The listing builds one solid part. Answer for the finished solid, in the listing's coordinates (mm). Face numbers are marked on the shaded views. Give positions to 0.01 mm unless a question says otherwise; leave off trailing zeros. Order: outer loops, then holes, each group sorted by start corner. A loop starts at its lowest first (then second) coordinate and runs counter-clockwise, first axis right, second up. Notation, with made-up numbers: (-28.5, 67) - (14.5, 67) arc R30 ccw to (14.5, 90) - close; hole circle Ø10 at (27.5, -1.5). An arc over 180 degrees is marked (long way). Answer as a JSON object with one key per item and string values. Group by question number.
Q1. The mould has two halves that part along Y. Classify the marked faces 1, 2, 3 and 4: released by +Y, released by -Y, zero draft, split by the parting line, or undercut.
Q2. Consider line 1 (Y direction, x = -70, z = -7); line 2 (Y direction, x = 17, z = 3); line 3 (Y direction, x = 7, z = 6.75) (1 decimal). Determine where each line is inside the solid, lowest interval first.
Q3. A cutting plane is placed at B-B, the plane y = -36. Give the vertices of the cut face in (x, z), and give its area (3 significant figures).
Q4. Given pin 1 (1.5 mm diameter, centred on y = 1.5, z = 0, fed in from +X); pin 2 (1.5 mm diameter, centred on x = -60.5, z = 5, fed in from -Y); pin 3 (1.5 mm diameter, centred on x = -41.5, z = -2, fed in from -Y), each flat-ended and moving along its own axis, determine where each tip first touches the part or whether it passes through.
Q5. A cutting plane is placed at A-A, the plane x = -70. Give the vertices of the cut face in (y, z).
Q6. A cutting plane is placed at C-C, the plane y = 0. Give the vertices of the cut face in (x, z).
Q7. A cutting plane is placed at D-D, the plane z = 5.5. Give the vertices of the cut face in (x, y) (3 decimals), and give its area (3 significant figures).
from build123d import *

# Parameters (mm, degrees)
SKETCH1_R           = 7.5
SKETCH1_R_2         = 15
BOSS_EXTRUDE1_DEPTH = 15


with BuildPart() as part:
    # Sketch1 → Boss-Extrude1 (new, symmetric)
    with BuildSketch(Plane.XY):
        with BuildLine():
            ThreePointArc((13.416465379, -41.130588018), (27.104825758, -44.598880973), (30.614150003, -30.920982406))
            ThreePointArc((30.614150003, -30.920982406), (23.463789692, -15.074619609), (19.905470006, 1.94223167))
            ThreePointArc((19.905470006, 1.94223167), (9.291872744, 17.710479974), (-9.714285714, 17.482352618))
            ThreePointArc((-9.714285714, 17.482352618), (-37.932007586, 8.122402385), (-67.619047619, 9.712418121))
            ThreePointArc((-67.619047619, 9.712418121), (-79.997392689, -0.228340587), (-67.178098245, -9.593584861))
            ThreePointArc((-67.178098245, -9.593584861), (-21.487956439, -11.580333122), (13.416465379, -41.130588018))
        make_face()
        with BuildLine():
            ThreePointArc((-18.010602512, 8.695872422), (-19.981112924, 0.868980041), (-18.697541465, -7.099432594))
            ThreePointArc((-18.697541465, -7.099432594), (-39.80648554, -2.386385888), (-61.287612025, -4.908594074))
            ThreePointArc((-61.287612025, -4.908594074), (-60.013800827, 0.525191469), (-61.850552891, 5.795387115))
            ThreePointArc((-61.850552891, 5.795387115), (-39.742227949, 4.398780735), (-18.010602512, 8.695872422))
        make_face(mode=Mode.SUBTRACT)
        with Locations((22, -36)):
            Circle(SKETCH1_R, mode=Mode.SUBTRACT)
        with BuildLine():
            ThreePointArc((17.591425152, -9.515343459), (20.794474813, -18.170038976), (24.906454326, -26.431691725))
            ThreePointArc((24.906454326, -26.431691725), (17.018206606, -27.32925986), (12.26998728, -33.692002498))
            ThreePointArc((12.26998728, -33.692002498), (7.22870194, -26.449040107), (1.246931193, -19.961091218))
            ThreePointArc((1.246931193, -19.961091218), (10.770298464, -16.852319454), (17.591425152, -9.515343459))
        make_face(mode=Mode.SUBTRACT)
        with Locations((-70, 0)):
            Circle(SKETCH1_R, mode=Mode.SUBTRACT)
        Circle(SKETCH1_R_2, mode=Mode.SUBTRACT)
    extrude(amount=BOSS_EXTRUDE1_DEPTH, both=True)


solid = part.part
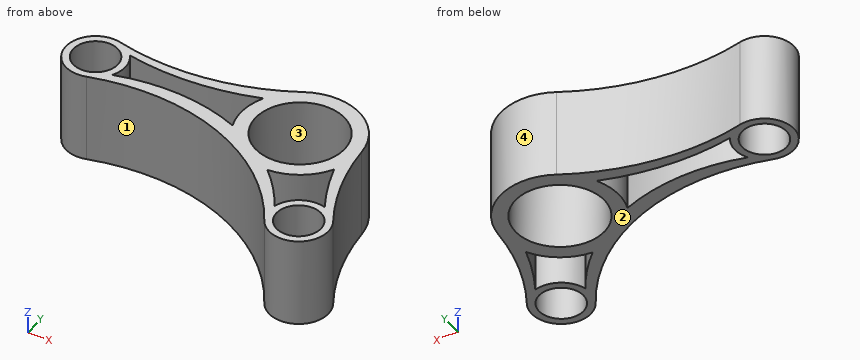
Reply:
{
 "1": {"face 1": "released by -Y", "face 2": "zero draft", "face 3": "undercut", "face 4": "released by +Y"},
 "2": {"line 1": "y = -10 to -7.5, 7.5 to 10", "line 2": "y = -44.66 to -41.59, -30.41 to -27.34, -10.54 to 10.54", "line 3": "y = -32.1 to -26.2, -18.7 to -13.3, 13.3 to 18.7"},
 "3": {"outline": "(10.04, -15) - (14.5, -15) - (14.5, 15) - (10.04, 15) - close; (29.5, -15) - (32, -15) - (32, 15) - (29.5, 15) - close", "area": "209 mm^2"},
 "4": {"pin 1": "stops at x = 20.03", "pin 2": "stops at y = -8.12", "pin 3": "stops at y = -7.02"},
 "5": {"outline": "(-10, -15) - (-7.5, -15) - (-7.5, 15) - (-10, 15) - close; (7.5, -15) - (10, -15) - (10, 15) - (7.5, 15) - close"},
 "6": {"outline": "(-80, -15) - (-77.5, -15) - (-77.5, 15) - (-80, 15) - close; (-62.5, -15) - (-60, -15) - (-60, 15) - (-62.5, 15) - close; (-20, -15) - (-15, -15) - (-15, 15) - (-20, 15) - close; (15, -15) - (20.12, -15) - (20.12, 15) - (15, 15) - close"},
 "7": {"outline": "(-67.619, 9.712) arc R10 ccw (long way) to (-67.178, -9.594) arc R70.663 cw to (13.416, -41.131) arc R10 ccw to (30.614, -30.921) arc R80 cw to (19.905, 1.942) arc R20 ccw to (-9.714, 17.482) arc R80 cw to start; hole circle Ø15 at (-70, 0); hole (-61.851, 5.795) arc R10 cw to (-61.288, -4.909) arc R64.57 cw to (-18.698, -7.099) arc R20 cw to (-18.011, 8.696) arc R86 cw to start; hole circle Ø30 at (0, 0); hole (1.247, -19.961) arc R64.57 cw to (12.27, -33.692) arc R10 cw to (24.906, -26.432) arc R86 cw to (17.591, -9.515) arc R20 cw to start; hole circle Ø15 at (22, -36)", "area": "1,390 mm^2"}
}
